Geometry: final body of the model. Coordinates: model frame, mm. Face numbers are marked on the shaded views. A direction names the side the tool comes from. Give positions to 0.01 mm unless a question says otherwise; leave off trailing zeros. Loops run counter-clockwise (first coordinate to the right, second up) from the corner with the lowest first, then second, coordinate; pieces in that order, holes last.
Autodesk Inventor part; units mm, degrees
ref_plane "YZ Plane" through (0, 0, 0) normal (1, 0, 0) x (0, 1, 0)
ref_plane "XZ Plane" through (0, 0, 0) normal (0, 1, 0) x (-1, 0, 0)
ref_plane "XY Plane" through (0, 0, 0) normal (0, 0, 1) x (1, 0, 0)
sketch "Rechteck" plane through (0, 0, 0) normal (0, 0, 1) x (1, 0, 0)
  line L0 (-5, 2) -> (5, 2)
  line L1 (5, 2) -> (5, -2)
  line L2 (5, -2) -> (-5, -2)
  line L3 (-5, -2) -> (-5, 2)
  point P0 (0, 0)
  dimension "d0" = 5
  dimension "d1" = 10
  dimension "d2" = 4
  dimension "d3" = 2
extrude "Extrusion1" add sketch "Rechteck" along normal blind 10
sketch "Kreis" plane through (-5, -2, 0) normal (0, -1, 0) x (1, 0, 0)
  circle A0 centre (5, 4) radius 2
  point P0 (5, 0)
  dimension "d6" = 4
extrude "Extrusion2" add sketch "Kreis" along normal blind 2
sketch "Dreieck" plane through (5, -2, 0) normal (1, 0, 0) x (0, 0, -1)
  line L0 (-5.0135, 2) -> (-7.0323, 0.8344)
  line L1 (-7.0323, 0.8344) -> (-7.0323, 3.1656)
  line L2 (-7.0323, 3.1656) -> (-5.0135, 2)
  point P0 (0, 2)
  point P1 (-6.3594, 2)
extrude "Extrusion3" add sketch "Dreieck" along normal blind 2
sketch "Pentagon" plane through (-5, 2, 0) normal (0, 1, 0) x (1, 0, 0)
  line L0 (5, -1.7907) -> (7.6131, -3.6893)
  line L1 (7.6131, -3.6893) -> (6.615, -6.7612)
  line L2 (6.615, -6.7612) -> (3.385, -6.7612)
  line L3 (3.385, -6.7612) -> (2.3869, -3.6893)
  line L4 (2.3869, -3.6893) -> (5, -1.7907)
  point P0 (5, 0)
  point P1 (5, -4.5383)
extrude "Extrusion4" add sketch "Pentagon" along normal blind 2
sketch "Hexagon" plane through (-5, -2, 0) normal (-1, 0, 0) x (0, 0, 1)
  line L0 (6.0229, 2) -> (5.5093, 1.1104)
  line L1 (5.5093, 1.1104) -> (4.4821, 1.1104)
  line L2 (4.4821, 1.1104) -> (3.9685, 2)
  line L3 (3.9685, 2) -> (4.4821, 2.8896)
  line L4 (4.4821, 2.8896) -> (5.5093, 2.8896)
  line L5 (5.5093, 2.8896) -> (6.0229, 2)
  point P0 (0, 2)
  point P1 (4.9957, 2)
extrude "Extrusion5" add sketch "Hexagon" along normal blind 2
sketch "Ellipse" plane through (0, 0, 10) normal (0, 0, 1) x (1, 0, 0)
  ellipse E0 centre (0, 0) end of major axis (3.8358, 0) minor radius 1.1104
sketch "Nase" plane through (0, 0, 0) normal (0, 0, -1) x (-1, 0, 0)
  line L0 (2.3535, 0) -> (-2.3535, 0) construction
  line L1 (2.3535, 0.5) -> (-2.3535, 0.5)
  line L2 (-2.3535, -0.5) -> (2.3535, -0.5)
  arc A0 (2.3535, -0.5) -> (2.3535, 0.5) centre (2.3535, 0) ccw
  arc A1 (-2.3535, 0.5) -> (-2.3535, -0.5) centre (-2.3535, 0) ccw
  point P0 (0, 0)
  dimension "d17" = 1
extrude "Extrusion7" add sketch "Nase" along normal blind 2
extrude "Extrusion8" add sketch "Ellipse" along normal blind 2
properties part number "Demo-Status-0.3"
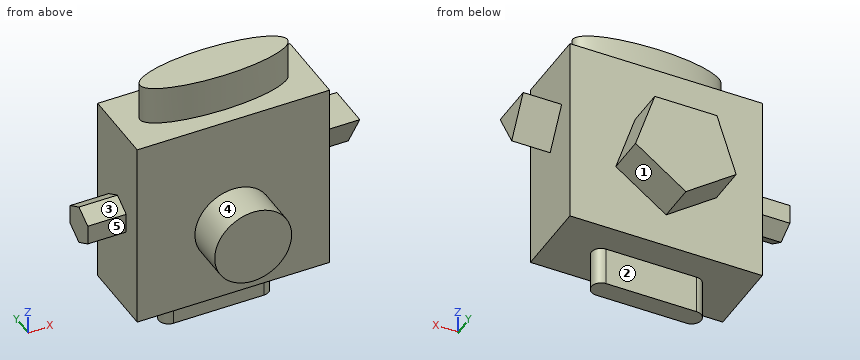
Item 1: Set-up query: the marked faces 1, 2, 3, 4 and 5. Return all of +Z, -Z, +X, -X, +Y, -Y with unobstructed straight access to the full face (end or side cutting, diameter ignored); none if empty.
Values follow:
face 1: -Z, +X, +Y
face 2: -Z, +X, -X, +Y
face 3: +Z, -X, -Y
face 4: -Y
face 5: +Z, -Z, -X, -Y
Item 2: Section query B-B on y = 3. Return loops of the section in (x, z) (3 decimals).
Values follow:
outline: (-2.613, 3.689) - (0, 1.791) - (2.613, 3.689) - (1.615, 6.761) - (-1.615, 6.761) - close
Item 3: Section query A-A on z = 2.5. Return loops of the section in (x, y), plus the area to 3 significant figures.
Values follow:
outline: (-5, -2) - (-1.32, -2) - (-1.32, -4) - (1.32, -4) - (1.32, -2) - (5, -2) - (5, 2) - (0.98, 2) - (0.98, 4) - (-0.98, 4) - (-0.98, 2) - (-5, 2) - close
area: 49.2 mm2
Item 4: Section query C-C on x = 4.5. Return loops of the section in (y, z), plus the area to 3 significant figures.
Values follow:
outline: (-2, 0) - (2, 0) - (2, 10) - (-2, 10) - close
area: 40.0 mm2
Item 5: Pin query (flat end, axial travel): pin 1 (5 mm diameter, centred on x = -2, z = 1.5, fed in from -Y); pin 2 (1.6 mm diameter, centred on x = 0.5, z = -0.5, fed in from -Y); pin 3 (0.5 mm diameter, centred on x = -6, z = 5, fed in from -Y); pin 4 (1.5 mm diameter, centred on x = 3, z = 9, fed in from +Y). Return the tip coordinate at first contact, or that it passes through.
Values follow:
pin 1: stops at y = -4
pin 2: stops at y = -2
pin 3: stops at y = -0.89
pin 4: stops at y = 2
Item 6: Section query D-D on z = 4.75. Return loops of the section in (x, y), plus the area to 3 significant figures.
Values follow:
outline: (-7, -0.89) - (-5, -0.89) - (-5, -2) - (-1.85, -2) - (-1.85, -4) - (1.85, -4) - (1.85, -2) - (5, -2) - (5, 2) - (2.27, 2) - (2.27, 4) - (-2.27, 4) - (-2.27, 2) - (-5, 2) - (-5, 0.89) - (-7, 0.89) - close
area: 60.0 mm2
Item 7: Ray query, probe 1 along X at (y, z) = (-1.5, 7); probe 2 along Y at (x, z) = (-0.25, 9.25); probe 3 along Z at (x, y) = (-1.5, -1.5). Return the intervals inside material, ascending.
Values follow:
probe 1: x = -5 to 5
probe 2: y = -2 to 2
probe 3: z = 0 to 10
